from build123d import *

# Parameters (mm, degrees)
CYLINDER_R     = 1.5
CYLINDER_DEPTH = 8
BOX_W          = 6
BOX_H          = 6
BOX_DEPTH      = 15


with BuildPart() as cylinder:
    # Cylinder → Cylinder (new body)
    with BuildSketch(Plane(origin=(3, 3, 7), x_dir=(1, 0, 0), z_dir=(0, 0, 1))):
        Circle(CYLINDER_R)
    extrude(amount=CYLINDER_DEPTH)


with BuildPart() as cut:
    # Box → Box (new body)
    with BuildSketch(Plane.XY):
        with Locations((3, 3)):
            Rectangle(BOX_W, BOX_H)
    extrude(amount=BOX_DEPTH)

    # Cut: cut Cylinder
    add(cylinder.part, mode=Mode.SUBTRACT)


solid = cut.part
Geometry: final body of the model. Coordinates: model frame, mm. Round coordinates to 2 decimals unless told otherwise and drop trailing zeros. Order: outer loops, then holes, each group sorted by start corner. A loop starts at its lowest first (then second) coordinate and runs counter-clockwise, first axis right, second up. Notation, with made-up numbers: (-17, 49) -> (31, 49) arc R8 cw to (31, 53) -> close; hole circle Ø3 at (-27, -5.5). An arc over 180 degrees is marked (long way). Put each result on its own line as item: value. Start each with the question number.
Q1. Section A-A on y = 3. Return the cut outline in (x, z).
Q2. Line query: probe 1 along Y at (x, z) = (2.9, 8.75); probe 2 along Y at (x, z) = (3.85, 11.25); probe 3 along Z at (x, y) = (3.4, 2.35). Output: solid intervals per line, ascending.
Q3. Section B-B on z = 8. Return the cut outline in (x, y).
Q4. Pull-direction query (Y, two-part tool) for faces 1 (the flat face through (3, 3, 7)), 2 (the cylindrical face through (3.69, 1.67, 10.94)), 3 (the flat face through (3, 6, 7)), 4 (the flat face through (6, 3, 7)); classes: +Y half, -Y half, draft (parallel to the pull), parting line (faces both ways), or undercut.
Ans:
1. outline: (0, 0) -> (6, 0) -> (6, 15) -> (4.5, 15) -> (4.5, 7) -> (1.5, 7) -> (1.5, 15) -> (0, 15) -> close
2. probe 1: y = 0 to 1.5, 4.5 to 6
2. probe 2: y = 0 to 1.76, 4.24 to 6
2. probe 3: z = 0 to 7
3. outline: (0, 0) -> (6, 0) -> (6, 6) -> (0, 6) -> close; hole circle Ø3 at (3, 3)
4. face 1: undercut
4. face 2: undercut
4. face 3: +Y half
4. face 4: draft
